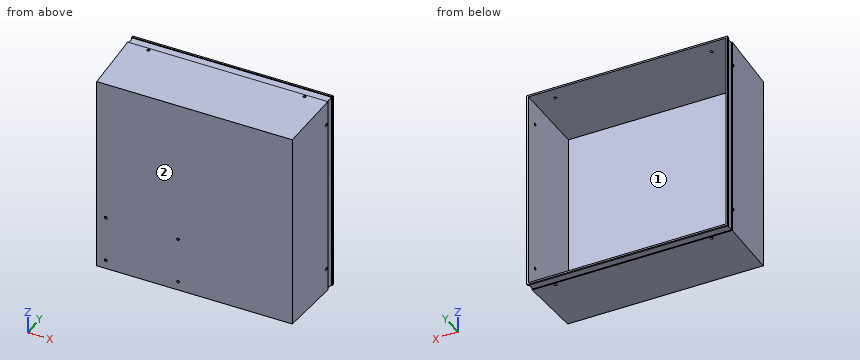
```python
from build123d import *

# Parameters (mm, degrees)
SKETCH1_W            = 238.1
SKETCH1_H            = 243.1
BOSS_EXTRUDE1_DEPTH  = 90
BOSS_EXTRUDE1_DRAFT  = -2
SHELL1_T             = -2
CUT_EXTRUDE7_DEPTH   = 291.651130828
CUT_EXTRUDE8_DEPTH   = 288.475472497
SKETCH10_R           = 1.7
CUT_EXTRUDE11_DEPTH  = 3
SKETCH11_R           = 1.7
CUT_EXTRUDE12_DEPTH  = 3
M3_CLEARANCE_HOLE2_D = 3.4


with BuildPart() as part:
    # Sketch1 → Boss-Extrude1 (with draft: the straight prism first)
    with BuildSketch(Plane(origin=(0, 0, 0), x_dir=(1, 0, 0), z_dir=(0, 1, 0))):
        Rectangle(SKETCH1_W, SKETCH1_H)
    extrude(amount=BOSS_EXTRUDE1_DEPTH)
    # Boss-Extrude1: the draft: its side faces are tilted about the plane it starts from
    boss_extrude1_sides = [part.faces().sort_by_distance(p)[0] for p in [
        (0, 45, 121.55),
        (119.05, 45, 0),
        (0, 45, -121.55),
        (-119.05, 45, 0),
    ]]
    draft(boss_extrude1_sides, Plane(origin=(0, 0, 0), x_dir=(1, 0, 0), z_dir=(0, 1, 0)), BOSS_EXTRUDE1_DRAFT)

    # Shell1
    shell1_openings = [part.faces().sort_by_distance(p)[0] for p in [
        (0, 90, 0),
    ]]
    offset(amount=SHELL1_T, openings=shell1_openings, kind=Kind.INTERSECTION)

    # Sketch6 → Cut-Extrude7 (cut, through all, along a direction that is not the sketch's normal)
    with BuildSketch(Plane(origin=(0, -4.239449692, 121.401955155), x_dir=(1, 0, 0), z_dir=(0, -0.03489949670250105, 0.9993908270190958))):
        Polygon((-122.123070261, 92.296892811), (-121.774287633, 82.302977128), (-120.773678831, 82.302977128), (-121.122461459, 92.296892811), align=None)
    cut_extrude7 = extrude(amount=-CUT_EXTRUDE7_DEPTH, dir=(0, 0, 1), mode=Mode.SUBTRACT)

    # Sketch7 → Cut-Extrude8 (cut, through all, along a direction that is not the sketch's normal)
    with BuildSketch(Plane(origin=(-118.905000092, -4.1522541, 0), x_dir=(0, 0, 1), z_dir=(-0.9993908270190958, -0.03489949670250105, 0))):
        Polygon((124.624288977, 92.209644069), (123.624288977, 92.209644069), (123.27550635, 82.215728386), (124.27550635, 82.215728386), align=None)
    cut_extrude8 = extrude(amount=-CUT_EXTRUDE8_DEPTH, dir=(-1, 0, 0), mode=Mode.SUBTRACT)

    # Mirror1: Cut-Extrude7 across plane
    add(cut_extrude7.mirror(Plane(origin=(0, 0, 0), x_dir=(0, 0, 1), z_dir=(1, 0, 0))), mode=Mode.SUBTRACT)

    # Mirror2: Cut-Extrude8 across plane
    add(cut_extrude8.mirror(Plane.XY), mode=Mode.SUBTRACT)

    # Sketch10 → Cut-Extrude11 (cut)
    with BuildSketch(Plane(origin=(0, -4.239449692, 121.401955155), x_dir=(1, 0, 0), z_dir=(0, -0.03489949670250105, 0.9993908270190958))):
        with Locations(Location((-95, 79.227051272, 0), (0, 0, 270))):
            Circle(SKETCH10_R)
        with Locations(Location((95, 79.227051272, 0), (0, 0, 270))):
            Circle(SKETCH10_R)
    cut_extrude11 = extrude(amount=-CUT_EXTRUDE11_DEPTH, mode=Mode.SUBTRACT)

    # Mirror3: Cut-Extrude11 across plane
    add(cut_extrude11.mirror(Plane.XY), mode=Mode.SUBTRACT)

    # Sketch11 → Cut-Extrude12 (cut)
    with BuildSketch(Plane(origin=(-118.905000092, -4.1522541, 0), x_dir=(0, 0, 1), z_dir=(-0.9993908270190958, -0.03489949670250105, 0))):
        with Locations(Location((-95, 79.13980253, 0), (0, 0, 270))):
            Circle(SKETCH11_R)
        with Locations(Location((95, 79.13980253, 0), (0, 0, 270))):
            Circle(SKETCH11_R)
    cut_extrude12 = extrude(amount=-CUT_EXTRUDE12_DEPTH, mode=Mode.SUBTRACT)

    # Mirror4: Cut-Extrude12 across plane
    add(cut_extrude12.mirror(Plane(origin=(0, 0, 0), x_dir=(0, 0, 1), z_dir=(1, 0, 0))), mode=Mode.SUBTRACT)

    # M3 Clearance Hole2 (through all)
    with Locations(Plane(origin=(0, 2, 0), x_dir=(1, 0, 0), z_dir=(0, 1, 0))):
        with Locations((-108.11862245, 54.61862245), (-108.11862245, 110.61862245), (-20.11862245, 110.61862245), (-20.11862245, 54.61862245)):
            Hole(M3_CLEARANCE_HOLE2_D / 2)


solid = part.part
```
Geometry: final body of the model. Coordinates: model frame, mm. Face numbers are marked on the shaded views. Coordinates: 2 decimals unless noted, no trailing zeros. Order: outer loops, then holes, each group sorted by start corner. A loop starts at its lowest first (then second) coordinate and runs counter-clockwise, first axis right, second up. Notation, with made-up numbers: (9, -9.5) -> (23, -9.5) arc R14 ccw to (23, -2.5) -> close; hole circle Ø11 at (-19.5, -12.75). An arc over 180 degrees is marked (long way). Write each question's results on one line, items separated by ' | '. Start each with the question number.
1) Material intervals for line 1 along X through (y, z) = (51, 59); line 2 along X through (y, z) = (12.5, -103.5); line 3 along Z through (x, y) = (-85.5, 60.5), sorted ascending.
2) Cut plane A-A, the plane x = 27. Output: boundary loops of the cut face in (y, z), and give its area (3 significant figures).
3) Cut plane C-C, the plane z = 52.5. Output: boundary loops of the cut face in (x, y), and give its area (3 significant figures).
4) Cut plane B-B, the plane y = 32. Output: boundary loops of the cut face in (x, z).
5) First-contact query: pin 1 (6 mm diameter, centred on x = 20, y = 24, fed in from -Z); pin 2 (1 mm diameter, centred on x = 43.5, z = -91, fed in from +Y); pin 3 (12 mm diameter, centred on y = 39.5, z = -13.5, fed in from +X); pin 4 (1 mm diameter, centred on x = 37.5, z = -69, fed in from -Y). Flat tips, straight axial feed; report the tip coordinate or a pass-through.
6) Mould query, pull axis Z, two halves, no side actions, for the marked faces 1 and 2. Classes: released by +Z, released by -Z, zero draft, split by the parting line, or undercut.
7) Cut plane D-D, the plane y = 69. Output: boundary loops of the cut face in (x, z), and give its area (3 significant figures).
Checks:
1) line 1: -120.83 to -118.83, 118.83 to 120.83 | line 2: -119.49 to -117.49, 117.49 to 119.49 | line 3: -123.66 to -121.66, 121.66 to 123.66
2) outline: (0, -121.55) -> (78.01, -124.27) -> (78.01, -123.28) -> (88, -123.62) -> (88, -124.62) -> (90, -124.69) -> (90, -122.69) -> (2, -119.62) -> (2, 119.62) -> (90, 122.69) -> (90, 124.69) -> (88, 124.62) -> (88, 123.62) -> (78.01, 123.28) -> (78.01, 124.27) -> (0, 121.55) -> close | area: 819 mm^2
3) outline: (-122.19, 90) -> (-122.12, 88) -> (-121.12, 88) -> (-120.77, 78.01) -> (-121.77, 78.01) -> (-119.05, 0) -> (119.05, 0) -> (121.77, 78.01) -> (120.77, 78.01) -> (121.12, 88) -> (122.12, 88) -> (122.19, 90) -> (120.19, 90) -> (117.12, 2) -> (-117.12, 2) -> (-120.19, 90) -> close | area: 809 mm^2
4) outline: (-120.17, -122.67) -> (120.17, -122.67) -> (120.17, 122.67) -> (-120.17, 122.67) -> close; hole (-118.17, -120.67) -> (118.17, -120.67) -> (118.17, 120.67) -> (-118.17, 120.67) -> close
5) pin 1: z = -122.49 | pin 2: y = 2 | pin 3: x = 120.64 | pin 4: y = 0
6) face 1: undercut | face 2: zero draft
7) outline: (-121.46, -123.96) -> (121.46, -123.96) -> (121.46, 123.96) -> (-121.46, 123.96) -> close; hole (-119.46, -121.96) -> (119.46, -121.96) -> (119.46, 121.96) -> (-119.46, 121.96) -> close | area: 1,950 mm^2
